```python
from build123d import *

# Parameters (mm, degrees)
ESBO_O1_R                = 12.425
ESBO_O1_R_2              = 1.2415
RESSALTO_EXTRUS_O1_DEPTH = 1.5
RESSALTO_EXTRUS_O2_START = -1
ESBO_O2_R                = 2.2
ESBO_O2_R_2              = 1.2415
RESSALTO_EXTRUS_O2_DEPTH = 1
RESSALTO_EXTRUS_O3_START = -100
ESBO_O3_R                = 1.2415
RESSALTO_EXTRUS_O3_DEPTH = 100
FILETE1_R                = 0.2


with BuildPart() as part:
    # Esboço1 → Ressalto-extrusão1 (new body)
    with BuildSketch(Plane.XY):
        Circle(ESBO_O1_R)
        Circle(ESBO_O1_R_2, mode=Mode.SUBTRACT)
    extrude(amount=RESSALTO_EXTRUS_O1_DEPTH)

    # Esboço2 → Ressalto-extrusão2 (add)
    with BuildSketch(Plane.XY.offset(RESSALTO_EXTRUS_O2_START)):
        Circle(ESBO_O2_R)
        Circle(ESBO_O2_R_2, mode=Mode.SUBTRACT)
    extrude(amount=RESSALTO_EXTRUS_O2_DEPTH)

    # Esboço3 → Ressalto-extrusão3 (add)
    with BuildSketch(Plane.XY.offset(16.5).offset(RESSALTO_EXTRUS_O3_START)):
        Circle(ESBO_O3_R)
    extrude(amount=RESSALTO_EXTRUS_O3_DEPTH)

    # Filete1
    filete1_edges = [part.edges().sort_by_distance(p)[0] for p in [
        (-1.2415, 0, -83.5),
        (-1.2415, 0, 16.5),
    ]]
    fillet(filete1_edges, radius=FILETE1_R)


solid = part.part
```
Can you work these out from the model? Positions are in its coordinate system, mm. A direction names the side the tool comes from. Round coordinates to 2 decimals unless told otherwise and drop trailing zeros. Loops run counter-clockwise (first coordinate to the right, second up) from the corner with the lowest first, then second, coordinate; pieces in that order, holes last. Notation, with made-up numbers: M 55,27 L 92,27 A21 ccw 92,53 Z; hole C -1.5,14 d9. An arc over 180 degrees is marked long. Answer as a JSON object with one key per item and string values. Group by question number.
Q1. Please list where these lines run through material, in increasing order: L1, parallel to Z at x = 6.5, y = -10.5; L2, parallel to X at y = -2.5, z = 1; L3, parallel to Y at x = -4.75, z = 1.
Q2. On a 3-axis mill with a long thin cutter (end or side, diameter ignored), from which of +Z, -Z, +X, -X, +Y, -Y can I reach the whole of each face in a straight line? I mean faces 1 (the cylindrical face through (-0.27, -1.21, 8.8)), 2 (the cylindrical face through (-0.27, -1.21, -42.73)), 3 (the flat face through (0, 0, 16.5)). Say none if no direction works.
Q3. Imagine slicing it at D-D, the plane x = 3.75. Please give me the cut outline in (y, z), then the cut area to 3 significant figures.
Q4. Will these pins go through, and if not, where does the flat tip stop? pin 1 (5 mm diameter, centred on x = -4, y = -3.5, fed in from +Z); pin 2 (8 mm diameter, centred on x = -7, y = 9.5, fed in from -Z); pin 3 (10 mm diameter, centred on x = -4, z = -17.5, fed in from -Y).
Q5. Imagine slicing it at C-C, the plane z = -62. Please give me the cut outline in (x, y), then the cut area to 3 significant figures.
Findings:
{
 "1": {"L1": "z = 0 to 1.5", "L2": "x = -12.17 to 12.17", "L3": "y = -11.48 to 11.48"},
 "2": {"face 1": "+Z", "face 2": "-Z", "face 3": "+Z, +X, -X, +Y, -Y"},
 "3": {"outline": "M -11.85,0 L 11.85,0 L 11.85,1.5 L -11.85,1.5 Z", "area": "35.5 mm2"},
 "4": {"pin 1": "stops at z = 1.5", "pin 2": "stops at z = 0", "pin 3": "stops at y = -1.24"},
 "5": {"outline": "C 0,0 d2.48", "area": "4.84 mm2"}
}
